The model under review builds one solid part; all positions refer to its coordinate system, in mm. Coordinates: 2 decimals unless noted, no trailing zeros. Write each loop counter-clockwise with the first axis right and the second up, starting at its lowest first coordinate (ties: lowest second). Pieces come first, ordered by that corner, then holes. Notation, with made-up numbers: (82, 48) - (107, 48) arc R33 cw to (107, 77) - close; hole circle Ø5 at (64, -4). An arc over 180 degrees is marked (long way). Put each result on its own line as item: value. Start each with the question number.
Item 1: For pin 1 (4 mm diameter, centred on x = 3.5, z = 3, fed in from +Y), flat-tipped, find the tip position at first contact; note if it passes through.
Item 2: Consider section A-A on x = 0. Give the boundary of the cut face in (y, z) (3 decimals), then the cut area to 3 significant figures.
Item 3: Consider section B-B on z = 0. Give the boundary of the cut face in (x, y) (3 decimals), then the cut area to 3 significant figures.
Item 4: Mouldability with a two-part tool opening along X and no side actions: class faces 1 (the face through (-10.16, 1, 0)), 2 (the face through (10.16, 1, 0)), 3 (the face through (0, 1, 10.16)), 4 (the face through (-7.874, 1.252, -2.48)) as pulls with the +X half, pulls with the -X half, needs draft (parallel to the pull), parting line crosses it, or undercut.
Item 5: To check wall thickness, follow L1, parallel to Z at x = 0, y = 1.7 (3 decimals); L2, parallel to X at y = 1.2, z = -3; L3, parallel to X at y = 1.8, z = 7.25. State the ranges of each line that lie inside material, in increasing order. Write a range as [from, to].
Item 6: Consider section C-C on y = 2.2. Give the boundary of the cut face in (x, z) (3 decimals).
Autodesk Inventor part; units mm, degrees
ref_plane "YZ Plane" through (0, 0, 0) normal (1, 0, 0) x (0, 1, 0)
ref_plane "XZ Plane" through (0, 0, 0) normal (0, 1, 0) x (-1, 0, 0)
ref_plane "XY Plane" through (0, 0, 0) normal (0, 0, 1) x (1, 0, 0)
sketch "Sketch1" plane through (0, 0, 0) normal (0, 1, 0) x (-1, 0, 0)
  circle A0 centre (0, 0) radius 8.255
  line L0 (10.16, -10.16) -> (-10.16, -10.16)
  line L1 (-10.16, -10.16) -> (-10.16, 10.16)
  line L2 (-10.16, 10.16) -> (10.16, 10.16)
  line L3 (10.16, 10.16) -> (10.16, -10.16)
  dimension "d0" = 16.51
  dimension "d4" = 20.32
  dimension "d5" = 10.16
  dimension "d6" = 20.32
  dimension "d7" = 10.16
extrude "Extrusion2" add sketch "Sketch1" along normal blind 2.54
properties part number "MarbleRingTest3"
Report:
1. pin 1: through
2. outline: (0, -10.16) - (2.54, -10.16) - (2.54, -8.255) - (0, -8.255) - close; (0, 8.255) - (2.54, 8.255) - (2.54, 10.16) - (0, 10.16) - close
2. area: 9.68 mm²
3. outline: (-10.16, 0) - (-8.255, 0) - (-8.255, 2.54) - (-10.16, 2.54) - close; (8.255, 0) - (10.16, 0) - (10.16, 2.54) - (8.255, 2.54) - close
3. area: 9.68 mm²
4. face 1: pulls with the -X half
4. face 2: pulls with the +X half
4. face 3: needs draft
4. face 4: undercut
5. L1: [-10.16, -8.255], [8.255, 10.16]
5. L2: [-10.16, -7.69], [7.69, 10.16]
5. L3: [-10.16, -3.95], [3.95, 10.16]
6. outline: (-10.16, -10.16) - (10.16, -10.16) - (10.16, 10.16) - (-10.16, 10.16) - close; hole circle Ø16.51 at (0, 0)
